Answer from the drawing. Dimensions are ordinates in mm from the lowest x, y and z of the part. Give positions to 0.01 mm unless a question says otherwise; leave off trailing zeros. Answer as CSV lines item,"result". Start each with the question number.
1) A straight line is drawn through the part: L1, parallel to Z at x = 260, y = 0.95. Find the intervals that lie inside material, in ascending order. Write a range as from..to.
2) Find section A-A (y = 1.2). State how many separate pieces and enclosed holes the cut face has, and give its area (3 significant figures).
3) A flat-ended cylindrical pin translates along its axis: pin 1 Ø1.8 at (x, z) = (4, 5.5) entering from -Y. Find the tip coordinate at first contact, or state that the pin passes through.
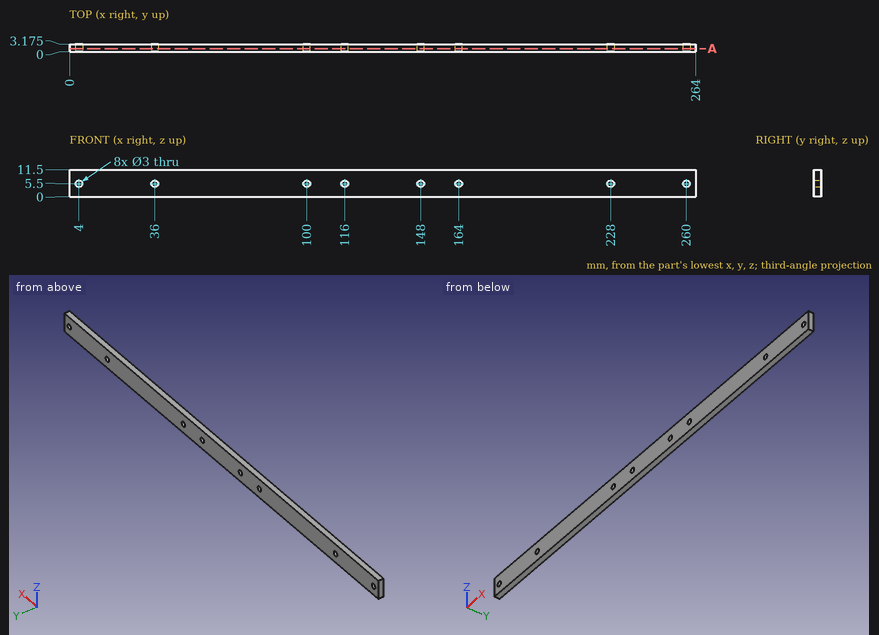
Findings below:
1,L1,"0..4, 7..11.5"
2,separate pieces,"1"
2,enclosed holes,"8"
2,area,"2,980 mm²"
3,pin 1,"through"
